Can you work these out from the model? Positions are in its coordinate system, mm. Face numbers are marked on the shaded views. A direction names the side the tool comes from. Round coordinates to 2 decimals unless told otherwise and drop trailing zeros. Loops run counter-clockwise (first coordinate to the right, second up) from the corner with the lowest first, then second, coordinate; pieces in that order, holes last. Notation, with made-up numbers: M 19.25,-21.5 L 58.25,-21.5 A21 ccw 58.25,-14.5 Z; hole C 8.5,3 d6. An arc over 180 degrees is marked long. Use a Markdown table: item, result. Add a question column.
```python
from build123d import *

# Parameters (mm, degrees)
SKETCH1_W           = 29
SKETCH1_H           = 26.5
BOSS_EXTRUDE1_DEPTH = 1
SKETCH2_R           = 1.1
CUT_EXTRUDE1_DEPTH  = 1
SKETCH3_W           = 27
SKETCH3_H           = 15
BOSS_EXTRUDE2_DEPTH = 1
SKETCH4_W           = 27
SKETCH4_H           = 19
BOSS_EXTRUDE3_DEPTH = 0.8
SKETCH5_R           = 0.75
CUT_EXTRUDE2_DEPTH  = 10.8


with BuildPart() as part:
    # Sketch1 → Boss-Extrude1 (new body)
    with BuildSketch(Plane(origin=(0, 0, 0), x_dir=(1, 0, 0), z_dir=(0, 1, 0))):
        with Locations((0, 0.5)):
            Rectangle(SKETCH1_W, SKETCH1_H)
    extrude(amount=BOSS_EXTRUDE1_DEPTH)

    # Sketch2 → Cut-Extrude1 (cut)
    with BuildSketch(Plane(origin=(0, 1, 0), x_dir=(1, 0, 0), z_dir=(0, 1, 0))):
        with Locations((-11.5, 12.25)):
            Circle(SKETCH2_R)
        with Locations((11.5, 12.25)):
            Circle(SKETCH2_R)
        with Locations((-11.5, -11.25)):
            Circle(SKETCH2_R)
        with Locations((11.5, -11.25)):
            Circle(SKETCH2_R)
    extrude(amount=-CUT_EXTRUDE1_DEPTH, mode=Mode.SUBTRACT)

    # Sketch3 → Boss-Extrude2 (add)
    with BuildSketch(Plane(origin=(0, 1, 0), x_dir=(1, 0, 0), z_dir=(0, 1, 0))):
        with Locations((0, 3)):
            Rectangle(SKETCH3_W, SKETCH3_H)
    extrude(amount=BOSS_EXTRUDE2_DEPTH)

    # Sketch4 → Boss-Extrude3 (add)
    with BuildSketch(Plane(origin=(0, 1, 0), x_dir=(1, 0, 0), z_dir=(0, 1, 0))):
        with Locations((0, 1)):
            Rectangle(SKETCH4_W, SKETCH4_H)
    extrude(amount=BOSS_EXTRUDE3_DEPTH)

    # Sketch5 → Cut-Extrude2 (cut)
    with BuildSketch(Plane(origin=(0, 1, 0), x_dir=(1, 0, 0), z_dir=(0, 1, 0))):
        with Locations((-1.27, 12.07364825)):
            Circle(SKETCH5_R)
        with Locations((1.27, 12.07364825)):
            Circle(SKETCH5_R)
        with Locations((3.81, 12.07364825)):
            Circle(SKETCH5_R)
        with Locations((-3.81, 12.07364825)):
            Circle(SKETCH5_R)
    extrude(amount=-CUT_EXTRUDE2_DEPTH, mode=Mode.SUBTRACT)


solid = part.part
```
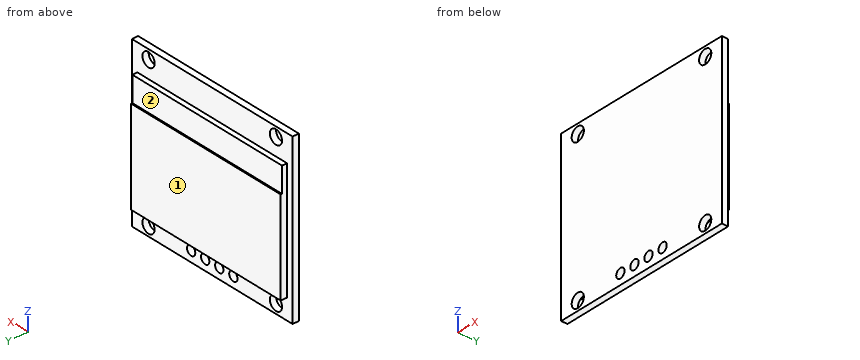
(1) On a 3-axis mill with a long thin cutter (end or side, diameter ignored), from which of +Z, -Z, +X, -X, +Y, -Y can I reach the whole of each face in a straight line? I mean the marked faces 1 and 2. Say none if no direction works.
(2) Suppose I cut it at B-B on x = -3.81. List the corners of the cut face in (y, z) for me.
(3) Suppose I cut it at C-C on z = 5.75. List the corners of the cut face in (x, y) for me.
(4) Suppose I cut it at D-D on x = -11.5. List the corners of the cut face in (y, z) for me.
(5) If I drill on probe 1 along X at (y, z) = (0.2, 11.25); probe 2 along Z at (x, y) = (11.5, 0.6); probe 3 along Y at (x, z) = (0.5, 5.75), over which ranges is the centre line in solid material (lowest first)? Write a range as [from, to].
(6) I'm going to push flat-ended pins straight in: pin 1 (0.5 mm diameter, centred on y = 1.5, z = -2.5, fed in from +X); pin 2 (0.8 mm diameter, centred on x = 4.5, y = 1.5, fed in from -Z); pin 3 (2.5 mm diameter, centred on x = 1.27, z = -12.07, fed in from +Y). Where does each tip first touch, or does it pass through?
(7) Suppose I cut it at A-A on z = 11.25. List the corners of the cut face in (x, y) for me.
Results below:
| question | item | result |
|---|---|---|
| 1 | face 1 | +Z, -Z, +X, -X, +Y |
| 1 | face 2 | +Z, +X, -X, +Y |
| 2 | outline | M 0,-13.75 L 1,-13.75 L 1,-12.82 L 0,-12.82 Z; M 0,-11.32 L 1,-11.32 L 1,-10.5 L 2,-10.5 L 2,4.5 L 1.8,4.5 L 1.8,8.5 L 1,8.5 L 1,12.75 L 0,12.75 Z |
| 3 | outline | M -14.5,0 L 14.5,0 L 14.5,1 L 13.5,1 L 13.5,1.8 L -13.5,1.8 L -13.5,1 L -14.5,1 Z |
| 4 | outline | M 0,-13.75 L 1,-13.75 L 1,-13.35 L 0,-13.35 Z; M 0,-11.15 L 1,-11.15 L 1,-10.5 L 2,-10.5 L 2,4.5 L 1.8,4.5 L 1.8,8.5 L 1,8.5 L 1,10.15 L 0,10.15 Z; M 0,12.35 L 1,12.35 L 1,12.75 L 0,12.75 Z |
| 5 | probe 1 | x = [-14.5, -12.6], [-10.4, 10.4], [12.6, 14.5] |
| 5 | probe 2 | z = [-13.75, -13.35], [-11.15, 10.15], [12.35, 12.75] |
| 5 | probe 3 | y = [0, 1.8] |
| 6 | pin 1 | stops at x = 13.5 |
| 6 | pin 2 | stops at z = -10.5 |
| 6 | pin 3 | stops at y = 1 |
| 7 | outline | M -14.5,0 L -12.6,0 L -12.6,1 L -14.5,1 Z; M -10.4,0 L 10.4,0 L 10.4,1 L -10.4,1 Z; M 12.6,0 L 14.5,0 L 14.5,1 L 12.6,1 Z |
